Here's the drawing with two shaded views (mm, measured from the low corner). I have some questions. Give positions to 0.01 mm unless a question says otherwise; leave off trailing zeros. Loops run counter-clockwise (first coordinate to the right, second up) from the corner with the lowest first, then second, coordinate; pieces in that order, holes last. Notation, with made-up numbers: (-26.5, -40) - (9.5, -40) arc R14 cw to (9.5, -34) - close; hole circle Ø6 at (12, 44). An arc over 180 degrees is marked (long way). Answer as a JSON object with one key per item and string values. Group by question number.
Item 1: Please list where these lines run through material, in increasing order: L1, parallel to X at y = 2.6, z = 33; L2, parallel to X at y = 0.6, z = 45; L3, parallel to Z at x = 48.5, y = 0.8.
Item 2: Suppose I cut it at A-A on z = 6. Write out the boundary of the cut face in (x, y).
Item 3: Will these pins go through, and if not, where does the flat tip stop? pin 1 (2 mm diameter, centred on x = 40, z = 13, fed in from -Y); pin 2 (1.2 mm diameter, centred on y = 0.5, z = 14, fed in from -X); pin 3 (0.5 mm diameter, centred on x = 2.5, z = 32.5, fed in from +Y); pin 4 (0.8 mm diameter, centred on y = 0.5, z = 20.5, fed in from +X).
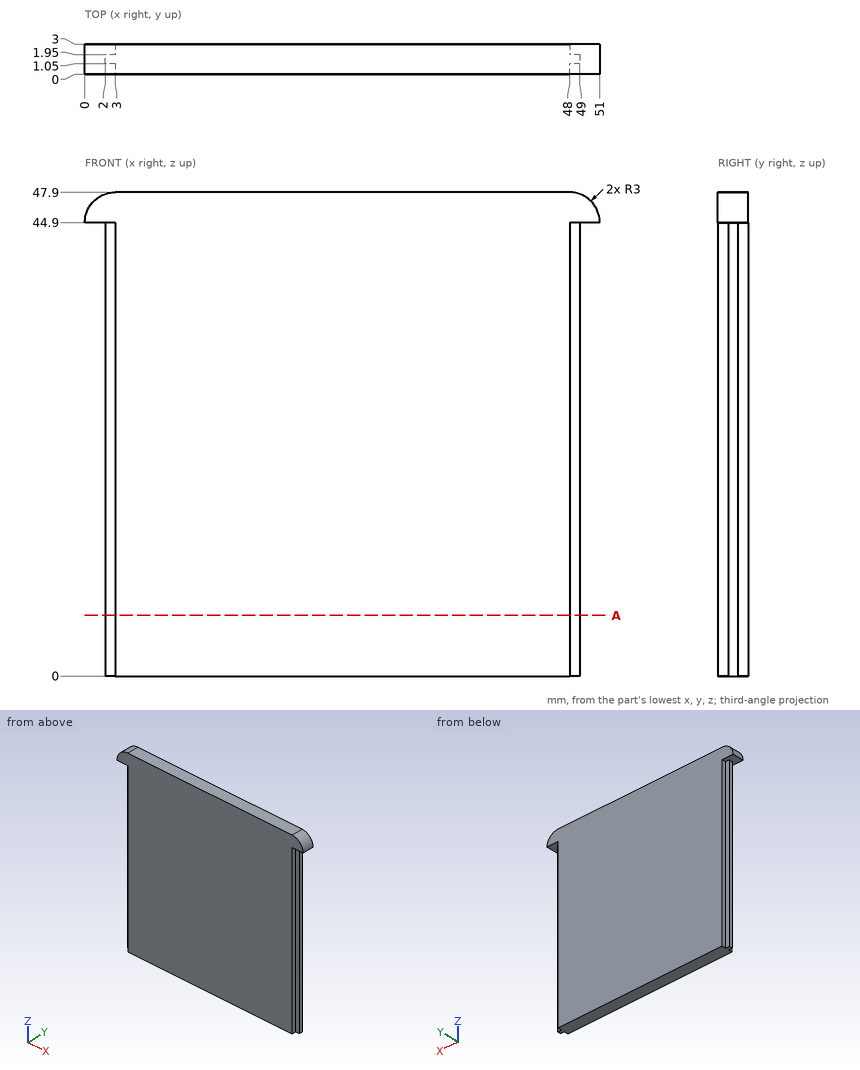
Worked out:
{
 "1": {"L1": "x = 3 to 48", "L2": "x = 0 to 51", "L3": "z = 44.9 to 47.86"},
 "2": {"outline": "(2, 1.05) - (3, 1.05) - (3, 0) - (48, 0) - (48, 1.05) - (49, 1.05) - (49, 1.95) - (48, 1.95) - (48, 3) - (3, 3) - (3, 1.95) - (2, 1.95) - close"},
 "3": {"pin 1": "stops at y = 0", "pin 2": "stops at x = 2", "pin 3": "stops at y = 1.95", "pin 4": "stops at x = 48"}
}
